Can you work these out from the drawing? Everything is in mm from the part's minimum corner. Round coordinates to 2 decimals unless told otherwise and drop trailing zeros. Write each loop counter-clockwise with the first axis right and the second up, starting at its lowest first coordinate (ties: lowest second). Pieces come first, ordered by that corner, then holes. Notation, with made-up numbers: (47, 79) -> (87, 79) arc R28 cw to (87, 113) -> close; hole circle Ø2 at (0, 84.25). An arc over 180 degrees is marked (long way). Put each result on its own line as item: value. Start each with the question number.
1. Suppose I cut it at B-B (x = 1.47). Please give me the cut outline in (y, z).
2. Suppose I cut it at A-A (x = 9.09). Please give me the cut outline in (y, z).
3. I need wall thicknesses on probe 1 along Y at (x, z) = (6.55, 0.85); probe 2 along X at (y, z) = (12.75, 0.5); probe 3 along X at (y, z) = (14.75, 0.2). Which ranges of each line are inside material? Lowest first, please. Write a range as from..to.
4. Suppose I cut it at C-C (z = 0.9). Count the separate pieces of the cut face and the enclosed holes in it, then the cut area to 3 significant figures.
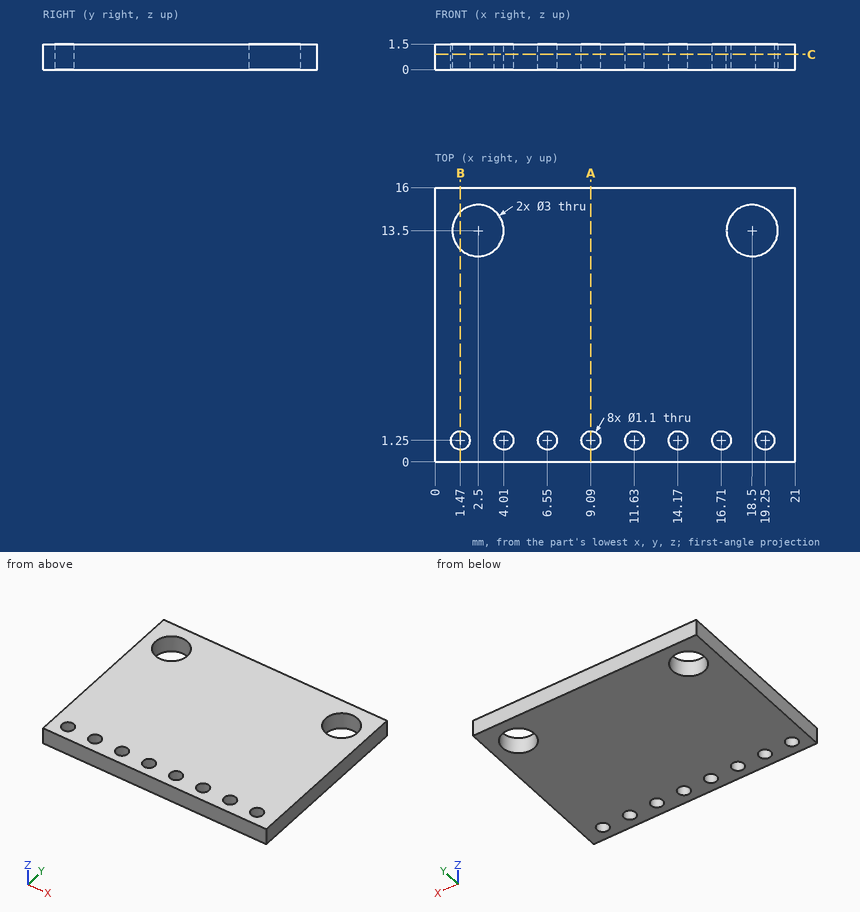
Verdict:
1. outline: (0, 0) -> (0.7, 0) -> (0.7, 1.5) -> (0, 1.5) -> close; (1.8, 0) -> (12.41, 0) -> (12.41, 1.5) -> (1.8, 1.5) -> close; (14.59, 0) -> (16, 0) -> (16, 1.5) -> (14.59, 1.5) -> close
2. outline: (0, 0) -> (0.7, 0) -> (0.7, 1.5) -> (0, 1.5) -> close; (1.8, 0) -> (16, 0) -> (16, 1.5) -> (1.8, 1.5) -> close
3. probe 1: y = 0..0.7, 1.8..16
3. probe 2: x = 0..1.2, 3.8..17.2, 19.8..21
3. probe 3: x = 0..1.67, 3.33..17.67, 19.33..21
4. separate pieces: 1
4. enclosed holes: 10
4. area: 314 mm^2
